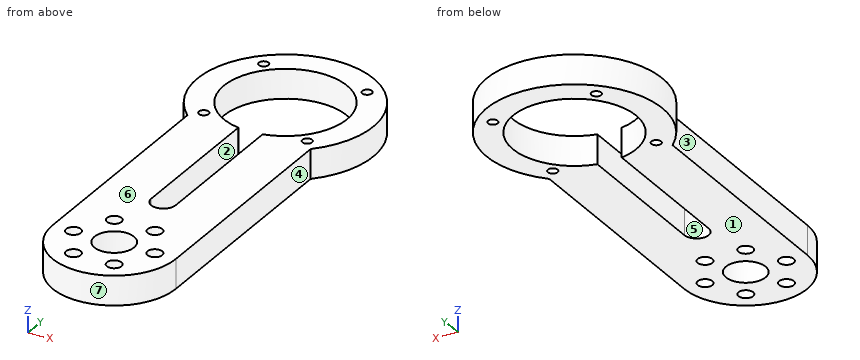
```python
from build123d import *

# Parameters (mm, degrees)
SKETCH1_R           = 6.75
SKETCH1_R_2         = 2.5
SKETCH1_R_3         = 1.65
SKETCH1_R_4         = 1.650080795
BOSS_EXTRUDE2_DEPTH = 10


with BuildPart() as part:
    # Sketch1 → Boss-Extrude2 (new body)
    with BuildSketch(Plane.XY):
        with BuildLine():
            Line((20.227196856, 25.327636264), (20.227196856, -53.948714213))
            ThreePointArc((20.227196856, -53.948714213), (-0.772803144, -74.948714213), (-21.772803144, -53.948714213))
            Line((-21.772803144, -53.948714213), (-21.772803144, 25.327636264))
            ThreePointArc((-21.772803144, 25.327636264), (-0.772803144, 76.751921549), (20.227196856, 25.327636264))
        make_face()
        with Locations((-0.772803144, -53.948714213)):
            Circle(SKETCH1_R, mode=Mode.SUBTRACT)
        with Locations((13.089121207, -53.948714213)):
            Circle(SKETCH1_R_2, mode=Mode.SUBTRACT)
        with Locations((6.158159031, -65.953492847)):
            Circle(SKETCH1_R_2, mode=Mode.SUBTRACT)
        with Locations((-7.703765319, -65.953492847)):
            Circle(SKETCH1_R_2, mode=Mode.SUBTRACT)
        with Locations((-14.634727495, -53.948714213)):
            Circle(SKETCH1_R_2, mode=Mode.SUBTRACT)
        with Locations((-7.703765319, -41.94393558)):
            Circle(SKETCH1_R_2, mode=Mode.SUBTRACT)
        with Locations((6.158159031, -41.94393558)):
            Circle(SKETCH1_R_2, mode=Mode.SUBTRACT)
        with Locations((-18.393960021, 64.373078426)):
            Circle(SKETCH1_R_3, mode=Mode.SUBTRACT)
        with Locations((-18.393960021, 29.130764673)):
            Circle(SKETCH1_R_3, mode=Mode.SUBTRACT)
        with Locations((16.848353733, 29.130764673)):
            Circle(SKETCH1_R_4, mode=Mode.SUBTRACT)
        with Locations((16.848353733, 64.373078426)):
            Circle(SKETCH1_R_3, mode=Mode.SUBTRACT)
        with BuildLine():
            Line((3.381188434, 25.751921549), (3.381188434, -25.007695686))
            ThreePointArc((3.381188434, -25.007695686), (-0.772803144, -29.161687264), (-4.926794722, -25.007695686))
            Line((-4.926794722, -25.007695686), (-4.926794722, 25.751921549))
            ThreePointArc((-4.926794722, 25.751921549), (-4.921699763, 25.957598174), (-4.906427385, 26.162770264))
            ThreePointArc((-4.906427385, 26.162770264), (-0.772803144, 67.751921549), (3.360821097, 26.162770264))
            ThreePointArc((3.360821097, 26.162770264), (3.376093476, 25.957598174), (3.381188434, 25.751921549))
        make_face(mode=Mode.SUBTRACT)
    extrude(amount=BOSS_EXTRUDE2_DEPTH)


solid = part.part
```
Verification items for the finished model (mm, model axes). Face numbers are marked on the shaded views. A direction names the side the tool comes from. Give positions to 0.01 mm unless a question says otherwise; leave off trailing zeros. Loops run counter-clockwise (first coordinate to the right, second up) from the corner with the lowest first, then second, coordinate; pieces in that order, holes last.
1. Mould release check, pull along Y, two halves, no side actions. Record for the marked faces 5, 6 and 7: released by +Y, released by -Y, zero draft, split by the parting line, or undercut.
2. Section check A-A, the plane y = 11.5. Enter the section's corners in (x, z).
3. Set-up check for the marked faces 1, 2, 3 and 4: record each of +Z, -Z, +X, -X, +Y, -Y from which the full face is reachable in a straight line by a thin tool's end or side.
4. Section check B-B, the plane x = -1. Enter the section's corners in (y, z).
5. Section check C-C, the plane z = 4. Count the separate pieces of the cut face and the enclosed holes in it, then the cut area to 3 significant figures.
6. Section check D-D, the plane y = 44.5. Enter the section's corners in (x, z), then the cut area to 3 significant figures.
7. Thickness scan on line 1 (X direction, y = -18, z = 5.25); line 2 (Y direction, x = -2, z = 2.25); line 3 (Y direction, x = -15, z = 4). Record the ranges inside material, lowest first.
8. Go/stop test with flat-tipped pins: pin 1 Ø3 at (x, z) = (14, 3.5) entering from -Y; pin 2 Ø4 at (x, z) = (-11, 2) entering from +Y; pin 3 Ø6 at (x, z) = (-3, 9) entering from -Y; pin 4 Ø4.5 at (x, y) = (-14.63, -53.95) entering from +Z. Record where each tip stops, or that it passes through.
Geometry says:
1. face 5: undercut
1. face 6: zero draft
1. face 7: released by -Y
2. outline: (-21.77, 0) - (-4.93, 0) - (-4.93, 10) - (-21.77, 10) - close; (3.38, 0) - (20.23, 0) - (20.23, 10) - (3.38, 10) - close
3. face 1: -Z, +X, -X, +Y, -Y
3. face 2: +Z, -Z
3. face 3: +Z, -Z, -X, -Y
3. face 4: +Z, -Z, +X, -Y
4. outline: (-74.95, 0) - (-60.69, 0) - (-60.69, 10) - (-74.95, 10) - close; (-47.2, 0) - (-29.16, 0) - (-29.16, 10) - (-47.2, 10) - close; (67.75, 0) - (76.75, 0) - (76.75, 10) - (67.75, 10) - close
5. separate pieces: 1
5. enclosed holes: 12
5. area: 4,470 mm2
6. outline: (-30.69, 0) - (-21.65, 0) - (-21.65, 10) - (-30.69, 10) - close; (20.11, 0) - (29.14, 0) - (29.14, 10) - (20.11, 10) - close
6. area: 181 mm2
7. line 1: x = -21.77 to -4.93, 3.38 to 20.23
7. line 2: y = -74.91 to -60.59, -47.31 to -28.98, 67.72 to 76.73
7. line 3: y = -69.39 to -56.42, -51.48 to 31.31, 62.2 to 73.16
8. pin 1: stops at y = -70.22
8. pin 2: stops at y = 75.6
8. pin 3: stops at y = -74.95
8. pin 4: passes through
